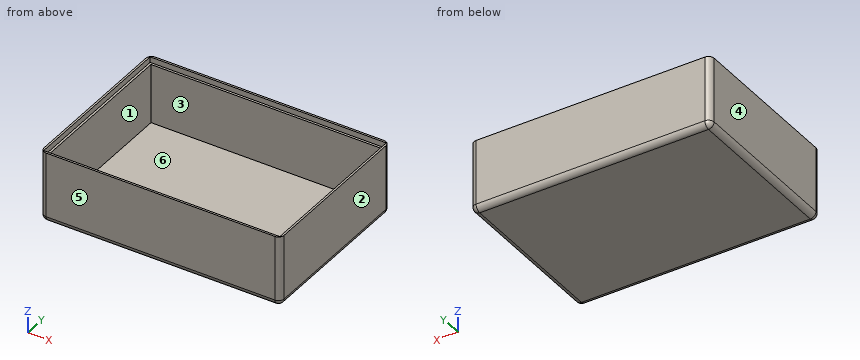
from build123d import *

# Parameters (mm, degrees)
SKETCH_1_W          = 85
SKETCH_1_H          = 60
EXTRUDE_1_DEPTH     = 25
SKETCH_2_W          = 82
SKETCH_2_H          = 57
CUT_EXTRUDE_1_DEPTH = 23
SKETCH_3_W          = 83.6
SKETCH_3_H          = 58.6
CUT_EXTRUDE_2_DEPTH = 2
FILLET_1_R          = 2


with BuildPart() as part:
    # 草图1 → 凸台-拉伸1 (new body)
    with BuildSketch(Plane.XY):
        with Locations((42.5, -30)):
            Rectangle(SKETCH_1_W, SKETCH_1_H)
    extrude(amount=EXTRUDE_1_DEPTH)

    # 草图2 → 切除-拉伸1 (cut)
    with BuildSketch(Plane.XY.offset(25)):
        with Locations((42.5, -30)):
            Rectangle(SKETCH_2_W, SKETCH_2_H)
    extrude(amount=-CUT_EXTRUDE_1_DEPTH, mode=Mode.SUBTRACT)

    # 草图3 → 切除-拉伸2 (cut)
    with BuildSketch(Plane.XY.offset(25)):
        with Locations((42.5, -30)):
            Rectangle(SKETCH_3_W, SKETCH_3_H)
    extrude(amount=-CUT_EXTRUDE_2_DEPTH, mode=Mode.SUBTRACT)

    # 圆角1
    fillet_1_edges = [part.edges().sort_by_distance(p)[0] for p in [
        (0, -30, 0),
        (42.5, -60, 0),
        (85, -30, 0),
        (42.5, 0, 0),
        (0, 0, 12.5),
        (0, -60, 12.5),
        (85, -60, 12.5),
        (85, 0, 12.5),
    ]]
    fillet(fillet_1_edges, radius=FILLET_1_R)


solid = part.part
Design review of the part built by this model. Coordinates are the model's own, in mm. Face numbers are marked on the shaded views. A direction names the side the tool comes from. Give positions to 0.01 mm unless a question says otherwise; leave off trailing zeros. Write each loop counter-clockwise with the first axis right and the second up, starting at its lowest first coordinate (ties: lowest second). Pieces come first, ordered by that corner, then holes. Notation, with made-up numbers: M 29,66.5 L 62,66.5 A35 ccw 62,102.5 Z; hole C 85,62 d9. An arc over 180 degrees is marked long. Return JSON: item names as keys, results as strings. Group by question number.
Item 1: Clearance check with a flat-ended pin moving along its axis: pin 1 Ø5 at (x, y) = (74.5, -42) entering from +Z. State where the tip first meets the part, or that it passes through.
Item 2: Take a section at B-B (y = -51.5). Give the boundary of the cut face in (x, z).
Item 3: Take a section at A-A (z = 5.5). Give the boundary of the cut face in (x, y), plus the area to 3 significant figures.
Item 4: Wall thickness on line 1 along X through (y, z) = (-45.5, 6.75); line 2 along Y through (x, z) = (27, 5); line 3 along X through (y, z) = (-45.5, 24): over which ranges is each line inside the solid? List them lowest first.
Item 5: Take a section at C-C (x = 31). Give the boundary of the cut face in (y, z).
Item 6: The part is to be moulded in two halves that separate along X. For the marked faces 3, 4, 5 and 6, say which applies: pulls with the +X half, pulls with the -X half, needs draft (parallel to the pull), parting line crosses it, or undercut.
Item 7: Tool access review of the marked faces 1 and 2: name each direction out of +Z, -Z, +X, -X, +Y, -Y from which nothing blocks a thin tool from reaching the whole face with its end or side.
Return value:
{
 "1": {"pin 1": "stops at z = 2"},
 "2": {"outline": "M 0,2 A2 ccw 2,0 L 83,0 A2 ccw 85,2 L 85,25 L 84.3,25 L 84.3,23 L 83.5,23 L 83.5,2 L 1.5,2 L 1.5,23 L 0.7,23 L 0.7,25 L 0,25 Z"},
 "3": {"outline": "M 0,-58 A2 ccw 2,-60 L 83,-60 A2 ccw 85,-58 L 85,-2 A2 ccw 83,0 L 2,0 A2 ccw 0,-2 Z; hole M 1.5,-58.5 L 83.5,-58.5 L 83.5,-1.5 L 1.5,-1.5 Z", "area": "423 mm2"},
 "4": {"line 1": "x = 0 to 1.5, 83.5 to 85", "line 2": "y = -60 to -58.5, -1.5 to 0", "line 3": "x = 0 to 0.7, 84.3 to 85"},
 "5": {"outline": "M -60,2 A2 ccw -58,0 L -2,0 A2 ccw 0,2 L 0,25 L -0.7,25 L -0.7,23 L -1.5,23 L -1.5,2 L -58.5,2 L -58.5,23 L -59.3,23 L -59.3,25 L -60,25 Z"},
 "6": {"face 3": "undercut", "face 4": "pulls with the -X half", "face 5": "needs draft", "face 6": "undercut"},
 "7": {"face 1": "+Z", "face 2": "+Z, -Z, +X, +Y, -Y"}
}
